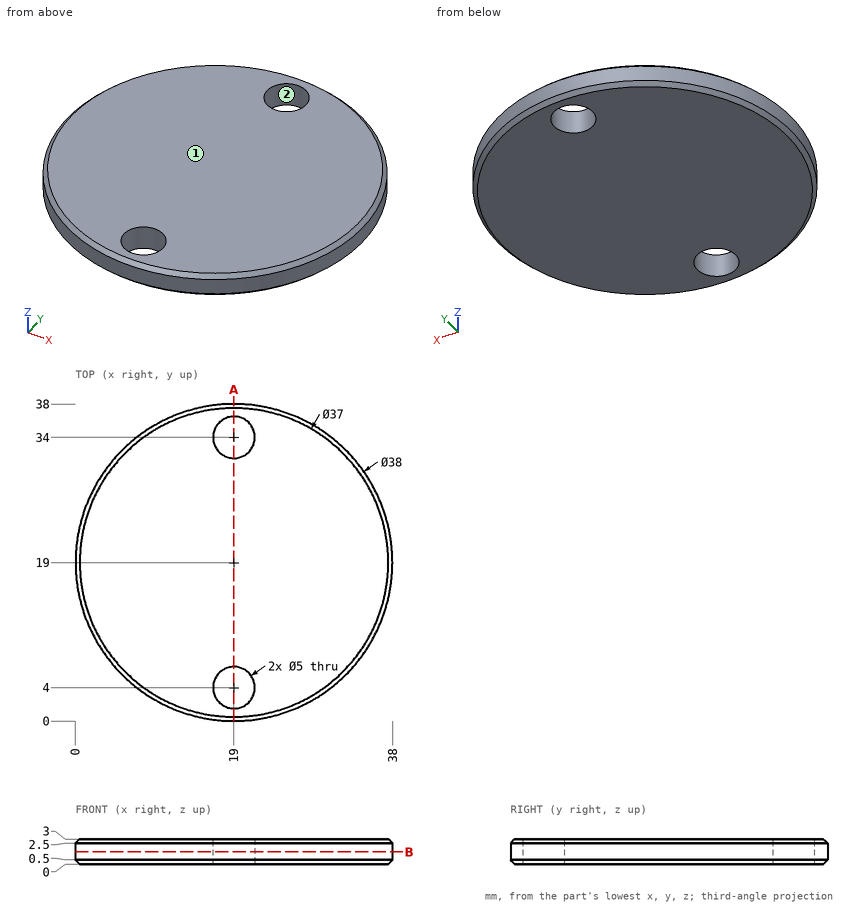
Verification items for this drawing (mm, ordinates from the low corner). Give positions to 0.01 mm unless a question says otherwise; leave off trailing zeros. Loops run counter-clockwise (first coordinate to the right, second up) from the corner with the lowest first, then second, coordinate; pieces in that order, holes last. Notation, with made-up numbers: M -10.5,-19 L 11.5,-19 A23 ccw 11.5,-1 Z; hole C 48,68 d10. An arc over 180 degrees is marked long. Return JSON: item names as keys, results as strings. Group by question number.
1. Mould release check, pull along X, two halves, no side actions. Record for the marked faces 1 and 2: released by +X, released by -X, zero draft, split by the parting line, or undercut.
2. Cross-section at A-A on x = 19. Record the boundary of the cut face in (y, z), plus the area to 3 significant figures.
3. Go/stop test with flat-tipped pins: pin 1 (1 mm diameter, centred on x = 32.5, z = 1.5, fed in from -Y); pin 2 (1 mm diameter, centred on x = 6, z = 1.5, fed in from -Y). Record where each tip stops, or that it passes through.
4. Cross-section at B-B on z = 1.45. Record the boundary of the cut face in (x, y), plus the area to 3 significant figures.
5. Thickness scan on L1, parallel to Y at x = 19, z = 1.3; L2, parallel to Y at x = 18.5, z = 2.3; L3, parallel to X at y = 18.5, z = 2.2. Record the ranges inside material, lowest first.
Return value:
{
 "1": {"face 1": "zero draft", "face 2": "undercut"},
 "2": {"outline": "M 0,0.5 L 0.5,0 L 1.5,0 L 1.5,3 L 0.5,3 L 0,2.5 Z; M 6.5,0 L 31.5,0 L 31.5,3 L 6.5,3 Z; M 36.5,0 L 37.5,0 L 38,0.5 L 38,2.5 L 37.5,3 L 36.5,3 Z", "area": "83.5 mm^2"},
 "3": {"pin 1": "y = 5.14", "pin 2": "y = 4.69"},
 "4": {"outline": "C 19,19 d38; hole C 19,4 d5; hole C 19,34 d5", "area": "1,090 mm^2"},
 "5": {"L1": "0 to 1.5, 6.5 to 31.5, 36.5 to 38", "L2": "0.01 to 1.55, 6.45 to 31.55, 36.45 to 37.99", "L3": "0.01 to 37.99"}
}
